The listing builds one solid part. Answer for the finished solid, in the listing's coordinates (mm). A direction names the side the tool comes from. Coordinates: 2 decimals unless noted, no trailing zeros. Loops run counter-clockwise (first coordinate to the right, second up) from the corner with the lowest first, then second, coordinate; pieces in that order, holes last. Notation, with made-up numbers: (-11.5, 72) - (25.5, 72) arc R21 cw to (25.5, 101) - close; hole circle Ø5 at (13, 39.5). An arc over 180 degrees is marked (long way). Return JSON: item names as keys, results as strings. Group by question number.
1. Section D-D (z = 75) is taken. Write down the section's boundary in (x, y).
2. Find the intervals of material crossed by line 1 along Z through (x, y) = (-11.5, 0.25); line 2 along X through (y, z) = (0.45, 75); line 3 along Y through (x, z) = (-12.5, 32), in increasing order.
3. Section C-C (y = 14) is taken. Write down the section's boundary in (x, z) (3 decimals).
4. Each of these flat-tipped pins is pushed along its axis until it touches: P1, Ø5, axis at x = -11.5, z = 10, coming from the -Y side; P2, Ø1, axis at x = -18, z = 124.5, coming from the +Y side. Where does it stop, or does it pass through?
5. The mould has two halves that part along Z. Classify faces 3 (the face through (-12.33, 0.28, 12.62)), 4 (the face through (-17, 3, 74)), 5 (the face through (-2.5, 8.9, 0)): pulls with the +Z half, pulls with the -Z half, needs draft (parallel to the pull), parting line crosses it, or undercut.
6. Section A-A (z = 35) is taken. Write down the section's boundary in (x, y).
7. Which of the six approach directions +Z, -Z, +X, -X, +Y, -Y give full straight-line access (tool end or side, diameter ignored) to faces 1 (the face through (-8.924, 0.703, 76.34)), 2 (the face through (-3, 14, 74))?
8. Section B-B (x = -11.5) is taken. Write down the section's boundary in (y, z), and give its area (3 significant figures).
```python
from build123d import *

# Parameters (mm, degrees)
BOSS_EXTRU_1_DEPTH                             = 150
FRAISAGE_POUR_VIS_T_TE_FRAIS_E_M41_D           = 4.5
FRAISAGE_POUR_VIS_T_TE_FRAIS_E_M41_DEPTH       = 25
FRAISAGE_POUR_VIS_T_TE_FRAIS_E_M41_CSINK_D     = 9.4
FRAISAGE_POUR_VIS_T_TE_FRAIS_E_M41_CSINK_ANGLE = 90
FRAISAGE_POUR_VIS_T_TE_FRAIS_E_M41_TIP         = 1.351936393
FRAISAGE_POUR_VIS_T_TE_FRAIS_E_M52_AT_COUNT    = 2
FRAISAGE_POUR_VIS_T_TE_FRAIS_E_M52_AT_PITCH    = 65
FRAISAGE_POUR_VIS_T_TE_FRAIS_E_M52_2_COUNT     = 2
FRAISAGE_POUR_VIS_T_TE_FRAIS_E_M52_2_PITCH     = 65


with BuildPart() as part:
    # Esquisse1 → Boss.-Extru.1 (new body)
    with BuildSketch(Plane.XY):
        Polygon((0, 25), (0, 0), (-20, 0), (-20, 3), (-3, 3), (-3, 25), align=None)
    extrude(amount=BOSS_EXTRU_1_DEPTH)

    # Fraisage pour vis à tête fraisée M41
    with Locations(Plane.ZY.offset(3)):
        with Locations((35, 14)):
            CounterSinkHole(FRAISAGE_POUR_VIS_T_TE_FRAIS_E_M41_D / 2, FRAISAGE_POUR_VIS_T_TE_FRAIS_E_M41_CSINK_D / 2, depth=FRAISAGE_POUR_VIS_T_TE_FRAIS_E_M41_DEPTH, counter_sink_angle=FRAISAGE_POUR_VIS_T_TE_FRAIS_E_M41_CSINK_ANGLE)
            with Locations((0, 0, -(FRAISAGE_POUR_VIS_T_TE_FRAIS_E_M41_DEPTH + FRAISAGE_POUR_VIS_T_TE_FRAIS_E_M41_TIP / 2))):  # 118° drill point
                Cone(0, FRAISAGE_POUR_VIS_T_TE_FRAIS_E_M41_D / 2, FRAISAGE_POUR_VIS_T_TE_FRAIS_E_M41_TIP, mode=Mode.SUBTRACT)

    # Esquisse6 → Trou taraudé M51 (revolve, cut)
    with BuildSketch(Plane(origin=(0, 14, 115), x_dir=(0, 0, -1), z_dir=(0, 1, 0))):
        Polygon((0, 0), (0, 3), (2.025, 3), (1.65, 2.625), (1.65, 0.375), (2.025, 0), align=None)
    revolve(axis=Axis((6.35, 14, 115), (-1, 0, 0)), mode=Mode.SUBTRACT)

    # Esquisse8 → Fraisage pour vis à tête fraisée M52 (revolve, cut)
    with BuildSketch(Plane(origin=(-11.5, 3, 75), x_dir=(0, 0, 1), z_dir=(1, 0, 0))):
        Polygon((0, 0), (0, 3), (2.75, 3), (2.75, 2.45), (5.2, 0), align=None)
    fraisage_pour_vis_t_te_frais_e_m52 = revolve(axis=Axis((-11.5, 9.35, 75), (0, -1, 0)), mode=Mode.SUBTRACT)

    # Fraisage pour vis à tête fraisée M52 at: Fraisage pour vis à tête fraisée M52 ×2
    with Locations(*[(0, 0, i * FRAISAGE_POUR_VIS_T_TE_FRAIS_E_M52_AT_PITCH) for i in range(1, FRAISAGE_POUR_VIS_T_TE_FRAIS_E_M52_AT_COUNT)]):
        add(fraisage_pour_vis_t_te_frais_e_m52, mode=Mode.SUBTRACT)

    # Fraisage pour vis _ t_te frais_e M52 2: Fraisage pour vis à tête fraisée M52 ×2
    with Locations(*[(0, 0, -i * FRAISAGE_POUR_VIS_T_TE_FRAIS_E_M52_2_PITCH) for i in range(1, FRAISAGE_POUR_VIS_T_TE_FRAIS_E_M52_2_COUNT)]):
        add(fraisage_pour_vis_t_te_frais_e_m52, mode=Mode.SUBTRACT)


solid = part.part
```
The answers:
{
 "1": {"outline": "(-20, 0) - (-14.25, 0) - (-14.25, 0.55) - (-16.7, 3) - (-20, 3) - close; (-8.75, 0) - (0, 0) - (0, 25) - (-3, 25) - (-3, 3) - (-6.3, 3) - (-8.75, 0.55) - close"},
 "2": {"line 1": "z = 0 to 7.25, 12.75 to 72.25, 77.75 to 137.25, 142.75 to 150", "line 2": "x = -20 to -14.25, -8.75 to 0", "line 3": "y = 0 to 3"},
 "3": {"outline": "(-3, 0) - (0, 0) - (0, 32.75) - (-0.55, 32.75) - (-3, 30.3) - close; (-3, 39.7) - (-0.55, 37.25) - (0, 37.25) - (0, 112.975) - (-0.375, 113.35) - (-2.625, 113.35) - (-3, 112.975) - close; (-3, 117.025) - (-2.625, 116.65) - (-0.375, 116.65) - (0, 117.025) - (0, 150) - (-3, 150) - close"},
 "4": {"P1": "passes through", "P2": "stops at y = 3"},
 "5": {"face 3": "undercut", "face 4": "needs draft", "face 5": "pulls with the -Z half"},
 "6": {"outline": "(-20, 0) - (0, 0) - (0, 11.75) - (-0.55, 11.75) - (-3, 9.3) - (-3, 3) - (-20, 3) - close; (-3, 18.7) - (-0.55, 16.25) - (0, 16.25) - (0, 25) - (-3, 25) - close"},
 "7": {"face 1": "+Y", "face 2": "+Z, -Z, -X, +Y"},
 "8": {"outline": "(0, 0) - (3, 0) - (3, 4.8) - (0.55, 7.25) - (0, 7.25) - close; (0, 12.75) - (0.55, 12.75) - (3, 15.2) - (3, 69.8) - (0.55, 72.25) - (0, 72.25) - close; (0, 77.75) - (0.55, 77.75) - (3, 80.2) - (3, 134.8) - (0.55, 137.25) - (0, 137.25) - close; (0, 142.75) - (0.55, 142.75) - (3, 145.2) - (3, 150) - (0, 150) - close", "area": "382 mm2"}
}
